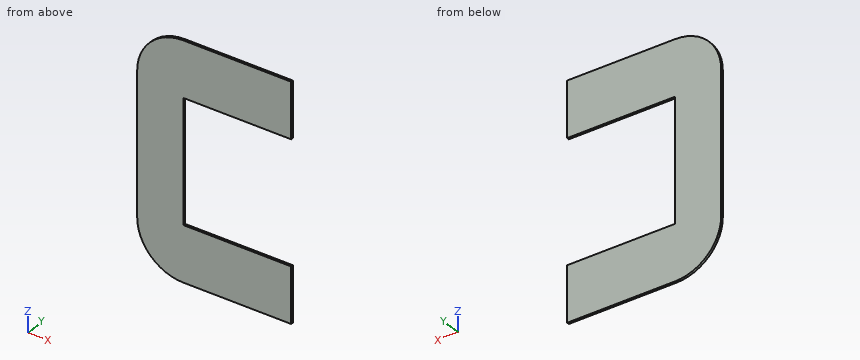
from build123d import *

# Parameters (mm, degrees)
SALIENTE_EXTRUIR1_DEPTH = 3
CROQUIS2_W              = 200
CROQUIS2_H              = 2.56
CORTAR_EXTRUIR1_DEPTH   = 10
CROQUIS3_W              = 140
CROQUIS3_H              = 160
CORTAR_EXTRUIR2_DEPTH   = 10
REDONDEO1_R             = 60


with BuildPart() as part:
    # Croquis1 → Saliente-Extruir1 (new body)
    with BuildSketch(Plane(origin=(0, 0, 0), x_dir=(1, 0, 0), z_dir=(0, 1, 0))):
        Polygon((-100, 155), (0, 155), (0, -155), (-100, -155), (-150, -155), (-200, -155), (-200, 155), (-150, 155), align=None)
    extrude(amount=SALIENTE_EXTRUIR1_DEPTH)

    # Croquis2 → Cortar-Extruir1 (cut)
    with BuildSketch(Plane(origin=(0, 3, 0), x_dir=(1, 0, 0), z_dir=(0, 1, 0))):
        with Locations((-100, 153.72)):
            Rectangle(CROQUIS2_W, CROQUIS2_H)
        with Locations((-100, -153.72)):
            Rectangle(CROQUIS2_W, CROQUIS2_H)
    extrude(amount=-CORTAR_EXTRUIR1_DEPTH, mode=Mode.SUBTRACT)

    # Croquis3 → Cortar-Extruir2 (cut)
    with BuildSketch(Plane(origin=(0, 3, 0), x_dir=(1, 0, 0), z_dir=(0, 1, 0))):
        with Locations((-70, 0)):
            Rectangle(CROQUIS3_W, CROQUIS3_H)
    extrude(amount=-CORTAR_EXTRUIR2_DEPTH, mode=Mode.SUBTRACT)

    # Redondeo1
    redondeo1_edges = [part.edges().sort_by_distance(p)[0] for p in [
        (-200, 1.5, -152.44),
        (-200, 1.5, 152.44),
    ]]
    fillet(redondeo1_edges, radius=REDONDEO1_R)


solid = part.part
Read the model definition and answer for the solid it produces. Units are mm, in the model's axes. Coordinates: 2 decimals unless noted, no trailing zeros. Order: outer loops, then holes, each group sorted by start corner. A loop starts at its lowest first (then second) coordinate and runs counter-clockwise, first axis right, second up. Notation, with made-up numbers: (81, 82) - (129, 82) arc R20 ccw to (129, 88) - close; hole circle Ø11 at (32.25, 5.25). An arc over 180 degrees is marked (long way). Use one line per item in the form item = value.
(1) Section A-A, the plane x = -109.5 is taken. Give the vertices of the cut face in (y, z).
Computed values:
outline = (0, -152.44) - (3, -152.44) - (3, -80) - (0, -80) - close; (0, 80) - (3, 80) - (3, 152.44) - (0, 152.44) - close
(2) Given pin 1 Ø6 at (x, z) = (-153, -53) entering from -Y, flat-ended and moving along its own axis, determine where the tip first touches the part or whether it passes through.
Computed values:
pin_1 = 0
(3) Section C-C, the plane z = -124.5 is taken. Give the vertices of the cut face in (x, y).
Computed values:
outline = (-190.72, 0) - (0, 0) - (0, 3) - (-190.72, 3) - close
(4) Straight lines are drawn through the part: L1, parallel to Z at x = -86.5, y = 2.35; L2, parallel to X at y = 0.8, z = -61.5; L3, parallel to X at y = 2.2, z = -94. For each, find the intervals that lie inside material, in ascending order.
Computed values:
L1 = -152.44 to -80, 80 to 152.44
L2 = -200 to -140
L3 = -199.98 to 0
(5) Section B-B, the plane y = 0.55 is taken. Give the vertices of the cut face in (x, z).
Computed values:
outline = (-200, -92.44) arc R60 ccw to (-140, -152.44) - (0, -152.44) - (0, -80) - (-140, -80) - (-140, 80) - (0, 80) - (0, 152.44) - (-140, 152.44) arc R60 ccw to (-200, 92.44) - close
(6) Section D-D, the plane x = -165 is taken. Give the vertices of the cut face in (y, z), then the cut area to 3 significant figures.
Computed values:
outline = (0, -146.98) - (3, -146.98) - (3, 146.98) - (0, 146.98) - close
area = 882 mm²
